from build123d import *

# Parameters (mm, degrees)
CROQUIS1_R              = 100
SALIENTE_EXTRUIR1_DEPTH = 3
CROQUIS3_R              = 110
CORTAR_EXTRUIR1_DEPTH   = 3
REDONDEO1_R             = 10
CORTAR_EXTRUIR2_DEPTH   = 142.453172607
CROQUIS6_W              = 10
CROQUIS6_H              = 50
CROQUIS6_W_2            = 30
CROQUIS6_H_2            = 10
CORTAR_EXTRUIR4_DEPTH   = 10
REDONDEO3_R             = 5
CROQUIS7_R              = 1.5
CORTAR_EXTRUIR5_DEPTH   = 142.453172607
CROQUIS8_R              = 1.5
CORTAR_EXTRUIR6_DEPTH   = 142.453172607


with BuildPart() as part:
    # Croquis1 → Saliente-Extruir1 (new body)
    with BuildSketch(Plane.XY):
        Circle(CROQUIS1_R)
    extrude(amount=SALIENTE_EXTRUIR1_DEPTH)

    # Croquis3 → Cortar-Extruir1 (cut)
    with BuildSketch(Plane.XY.offset(3)):
        with Locations((190, 0)):
            Circle(CROQUIS3_R)
    extrude(amount=-CORTAR_EXTRUIR1_DEPTH, mode=Mode.SUBTRACT)

    # Redondeo1
    redondeo1_edges = [part.edges().sort_by_distance(p)[0] for p in [
        (89.473684211, -44.659375654, 1.5),
        (89.473684211, 44.659375654, 1.5),
    ]]
    fillet(redondeo1_edges, radius=REDONDEO1_R)

    # Croquis4 → Cortar-Extruir2 (cut, through all)
    with BuildSketch(Plane.XY.offset(3)):
        Polygon((-57.629202667, -83.792153571), (-83.792153571, -57.629202667), (-68.235804385, -42.072853481), (-42.072853481, -68.235804385), align=None)
        Polygon((-57.629202667, 83.792153571), (-42.072853481, 68.235804385), (-68.235804385, 42.072853481), (-83.792153571, 57.629202667), align=None)
        Polygon((83.792153571, 57.629202667), (68.235804385, 42.072853481), (42.072853481, 68.235804385), (57.629202667, 83.792153571), align=None)
        Polygon((57.629202667, -83.792153571), (42.072853481, -68.235804385), (68.235804385, -42.072853481), (83.792153571, -57.629202667), align=None)
    extrude(amount=-CORTAR_EXTRUIR2_DEPTH, mode=Mode.SUBTRACT)

    # Croquis6 → Cortar-Extruir4 (cut)
    with BuildSketch(Plane.XY.offset(3)):
        with Locations((-68.235804385, 0)):
            Rectangle(CROQUIS6_W, CROQUIS6_H)
        with Locations((0, 73.24)):
            Rectangle(CROQUIS6_W_2, CROQUIS6_H_2)
        with Locations((0, -73.24)):
            Rectangle(CROQUIS6_W_2, CROQUIS6_H_2)
    extrude(amount=-CORTAR_EXTRUIR4_DEPTH, mode=Mode.SUBTRACT)

    # Redondeo3
    redondeo3_edges = [part.edges().sort_by_distance(p)[0] for p in [
        (15, -78.24, 1.5),
        (-15, -78.24, 1.5),
        (15, -68.24, 1.5),
        (-15, -68.24, 1.5),
        (-73.235804385, -25, 1.5),
        (-63.235804385, -25, 1.5),
        (-73.235804385, 25, 1.5),
        (-63.235804385, 25, 1.5),
        (-15, 68.24, 1.5),
        (15, 68.24, 1.5),
        (-15, 78.24, 1.5),
        (15, 78.24, 1.5),
    ]]
    fillet(redondeo3_edges, radius=REDONDEO3_R - 0.0001)  # a hair under: the kernel refuses the full size

    # Croquis7 → Cortar-Extruir5 (cut, through all)
    with BuildSketch(Plane(origin=(0, 0, 0), x_dir=(-1, 0, 0), z_dir=(0, 0, -1))):
        with Locations((37.565, -24.17)):
            Circle(CROQUIS7_R)
        with Locations((-37.565, -24.17)):
            Circle(CROQUIS7_R)
        with Locations((-45.065, 24.17)):
            Circle(CROQUIS7_R)
        with Locations((37.565, 24.17)):
            Circle(CROQUIS7_R)
        with Locations((-14.06559482, 19.297497716)):
            Circle(CROQUIS7_R)
        with Locations((-14.061195262, -8.714642909)):
            Circle(CROQUIS7_R)
    extrude(amount=-CORTAR_EXTRUIR5_DEPTH, mode=Mode.SUBTRACT)

    # Croquis8 → Cortar-Extruir6 (cut, through all)
    with BuildSketch(Plane(origin=(0, 0, 0), x_dir=(-1, 0, 0), z_dir=(0, 0, -1))):
        with Locations((-20.32, 35)):
            Circle(CROQUIS8_R)
        with Locations((20.32, 35)):
            Circle(CROQUIS8_R)
        with Locations(Location((20.32, -35, 0), (0, 0, 180))):
            Circle(CROQUIS8_R)
        with Locations(Location((-20.32, -35, 0), (0, 0, 180))):
            Circle(CROQUIS8_R)
    extrude(amount=-CORTAR_EXTRUIR6_DEPTH, mode=Mode.SUBTRACT)


solid = part.part
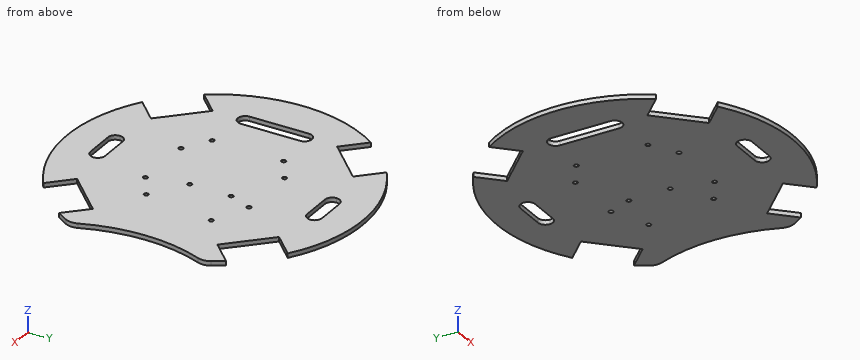
Can you work these out from the model? Positions are in its coordinate system, mm. Coordinates: 2 decimals unless noted, no trailing zeros. Write each loop counter-clockwise with the first axis right and the second up, starting at its lowest first coordinate (ties: lowest second). Pieces come first, ordered by that corner, then holes. Notation, with made-up numbers: (2.5, 39) - (26.5, 39) arc R22 ccw to (26.5, 47) - close; hole circle Ø5 at (43.25, -34). An arc over 180 degrees is marked (long way). Return JSON: item names as keys, results as strings. Group by question number.
Item 1: If we section it at C-C (z = 0.55): Count the separate pieces of the cut face and the enclosed holes in it, then the cut area to 3 significant figures.
Item 2: If we section it at A-A (y = 15): Write out the boundary of the cut face in (x, z).
Item 3: Please list where these lines run through material, in increasing order: probe 1 along Y at (x, z) = (-0.5, 0.75); probe 2 along Y at (x, z) = (-50.5, 1.2); probe 3 along X at (y, z) = (-24, 1.15).
Item 4: If we section it at D-D (x = -46.5): Write out the boundary of the cut face in (y, z).
Item 5: I'm going to push flat-ended pins straight in: pin 1 Ø1.5 at (y, z) = (-7, 1) entering from -X; pin 2 Ø1.5 at (x, z) = (-1, 0.5) entering from -Y; pin 3 Ø1.5 at (y, z) = (-35.5, 2.5) entering from -X. Where does each tip first touch, or does it pass through?
Item 6: If we section it at B-B (x = 2.5): Write out the boundary of the cut face in (y, z), then the cut area to 3 significant figures.
Return value:
{
 "1": {"separate pieces": "1", "enclosed holes": "13", "area": "25,900 mm^2"},
 "2": {"outline": "(-98.87, 0) - (-73.24, 0) - (-73.24, 3) - (-98.87, 3) - close; (-63.24, 0) - (81.03, 0) - (81.03, 3) - (-63.24, 3) - close"},
 "3": {"probe 1": "y = -100 to -78.24, -68.24 to 68.24, 78.24 to 100", "probe 2": "y = -86.31 to -76.66, -59.81 to 59.81, 76.66 to 86.31", "probe 3": "x = -97.08 to -71.24, -65.24 to -39.06, -36.07 to 36.07, 39.06 to 82.65"},
 "4": {"outline": "(-88.53, 0) - (-72.66, 0) - (-72.66, 3) - (-88.53, 3) - close; (-63.81, 0) - (63.81, 0) - (63.81, 3) - (-63.81, 3) - close; (72.66, 0) - (88.53, 0) - (88.53, 3) - (72.66, 3) - close"},
 "5": {"pin 1": "stops at x = -99.8", "pin 2": "stops at y = -100", "pin 3": "stops at x = -93.77"},
 "6": {"outline": "(-99.97, 0) - (-78.24, 0) - (-78.24, 3) - (-99.97, 3) - close; (-68.24, 0) - (68.24, 0) - (68.24, 3) - (-68.24, 3) - close; (78.24, 0) - (99.97, 0) - (99.97, 3) - (78.24, 3) - close", "area": "540 mm^2"}
}
